The model under review builds one solid part; all positions refer to its coordinate system, in mm. A direction names the side the tool comes from. Round coordinates to 2 decimals unless told otherwise and drop trailing zeros. Write each loop counter-clockwise with the first axis right and the second up, starting at its lowest first coordinate (ties: lowest second). Pieces come first, ordered by that corner, then holes.
Item 1: Add section B-B (z = -8). State how many separate pieces and enclosed holes the cut face has, plus the area to 3 significant figures.
Item 2: Add section A-A (y = 100). Give the boundary of the cut face in (x, z).
Item 3: Clearance check with flat-ended pins moving along their axes: pin 1 Ø4.5 at (y, z) = (12, -8) entering from +X; pin 2 Ø1 at (x, y) = (10.5, 57) entering from -Z. State where each tip first meets the part, or that it passes through.
Item 4: To check wall thickness, follow L1, parallel to X at y = 92.5, z = -3; L2, parallel to Z at x = 4.75, y = 101; L3, parallel to X at y = 36.5, z = -1.75. State the ranges of each line that lie inside material, in increasing order.
Item 5: Add section C-C (x = 4). Give the boundary of the cut face in (y, z).
Item 6: Draft analysis for pull direction Y (two halves, no side actions). For faces 3 (the face through (1, 42, -8)), 4 (the face through (2.5, 67, -5)), 5 (the face through (8, 70, -1)), state which applies: +Y half, -Y half, draft (parallel to the pull), parting line (faces both ways), or undercut.
Item 7: Machinability: for faces 1 (the face through (6, 67, -2.5)), 2 (the face through (1, 102, -8)), which of the approach directions +Z, -Z, +X, -X, +Y, -Y give a long, thin tool a straight path to every point of the face, cutting with its end or side? Answer none if there is none.
```python
from build123d import *

# Parameters (mm, degrees)
SKETCH1_W                = 136
SKETCH1_H                = 12
BOSS_EXTRUDE1_DEPTH      = 12
SKETCH2_W                = 9.5
SKETCH2_H                = 9.5
CUT_EXTRUDE1_DEPTH       = 138.054733592
F_4_0_4_DIAMETER_HOLE1_D = 4
F_4_0_4_DIAMETER_HOLE2_D = 4


with BuildPart() as part:
    # Sketch1 → Boss-Extrude1 (new body)
    with BuildSketch(Plane(origin=(0, 0, 0), x_dir=(0, -1, 0), z_dir=(-1, 0, 0))):
        with Locations((-68, -6)):
            Rectangle(SKETCH1_W, SKETCH1_H)
    extrude(amount=-BOSS_EXTRUDE1_DEPTH)

    # Sketch2 → Cut-Extrude1 (cut, through all)
    with BuildSketch(Plane.XZ):
        with Locations((7.25, -7.25)):
            Rectangle(SKETCH2_W, SKETCH2_H)
    extrude(amount=-CUT_EXTRUDE1_DEPTH, mode=Mode.SUBTRACT)

    # Ø4.0 (4) Diameter Hole1 (through all)
    with Locations(Plane(origin=(0, 0, -2.5), x_dir=(-1, 0, 0), z_dir=(0, 0, -1))):
        with Locations((-8, 4), (-8, 12), (-8, 20), (-8, 28), (-8, 36), (-8, 44), (-8, 52), (-8, 60), (-8, 68), (-8, 76), (-8, 84), (-8, 92), (-8, 100), (-8, 108), (-8, 116), (-8, 124), (-8, 132)):
            Hole(F_4_0_4_DIAMETER_HOLE1_D / 2)

    # Ø4.0 (4) Diameter Hole2 (through all)
    with Locations(Plane(origin=(2.5, 0, 0), x_dir=(0, 0, -1), z_dir=(1, 0, 0))):
        with Locations((8, 12), (8, 4), (8, 20), (8, 28), (8, 36), (8, 44), (8, 52), (8, 60), (8, 68), (8, 76), (8, 84), (8, 92), (8, 100), (8, 108), (8, 116), (8, 124), (8, 132)):
            Hole(F_4_0_4_DIAMETER_HOLE2_D / 2)


solid = part.part
```
Numbers:
1. separate pieces: 18
1. enclosed holes: 0
1. area: 170 mm2
2. outline: (0, -12) - (2.5, -12) - (2.5, -10) - (0, -10) - close; (0, -6) - (2.5, -6) - (2.5, -2.5) - (6, -2.5) - (6, 0) - (0, 0) - close; (10, -2.5) - (12, -2.5) - (12, 0) - (10, 0) - close
3. pin 1: stops at x = 2.5
3. pin 2: stops at z = -2.5
4. L1: x = 0 to 2.5
4. L2: z = -2.5 to 0
4. L3: x = 0 to 6.06, 9.94 to 12
5. outline: (0, -2.5) - (136, -2.5) - (136, 0) - (0, 0) - close
6. face 3: undercut
6. face 4: draft
6. face 5: undercut
7. face 1: -Z, +X, +Y, -Y
7. face 2: +X, -X
